```python
from build123d import *

# Parameters (mm, degrees)
F1_R     = 1.6
F1_W     = 26.4
F1_H     = 5
F1_W_2   = 20
F1_W_3   = 5
F2_DEPTH = 5


with BuildPart() as f2:
    # F1 (on Right) → F2 (new body)
    with BuildSketch(Plane.YZ):
        with BuildLine():
            Line((0, 5), (0, 0))
            Line((0, 0), (33.5, 0))
            Line((33.5, 0), (33.5, -5))
            Line((33.5, -5), (38.5, -5))
            Line((38.5, -5), (38.5, 0))
            Line((38.5, 0), (47, 0))
            Line((47, 0), (47, 2))
            Line((47, 2), (45.75, 2))
            Line((45.75, 2), (45.75, 5))
            Line((45.75, 5), (47, 5))
            Line((47, 5), (47, 6))
            Line((47, 6), (50, 6))
            Line((50, 6), (50, 5))
            Line((50, 5), (51.25, 5))
            Line((51.25, 5), (51.25, 2))
            Line((51.25, 2), (50, 2))
            Line((50, 2), (50, 0))
            Line((50, 0), (58.5, 0))
            Line((58.5, 0), (58.5, -5))
            Line((58.5, -5), (63.5, -5))
            Line((63.5, -5), (63.5, 0))
            Line((63.5, 0), (97, 0))
            Line((97, 0), (118.2132034356, -21.2132034356))
            Line((118.2132034356, -21.2132034356), (125.2842712475, -28.2842712475))
            Line((125.2842712475, -28.2842712475), (131.2239682094, -34.2239682094))
            Line((131.2239682094, -34.2239682094), (132.9917351624, -32.4562012565))
            Line((132.9917351624, -32.4562012565), (132.178562364, -31.6430284581))
            Line((132.178562364, -31.6430284581), (133.946329317, -29.8752615051))
            Line((133.946329317, -29.8752615051), (135.8908729653, -31.8198051534))
            Line((135.8908729653, -31.8198051534), (137.8354166135, -33.7643488017))
            Line((137.8354166135, -33.7643488017), (136.0676496606, -35.5321157546))
            Line((136.0676496606, -35.5321157546), (135.2544768622, -34.7189429563))
            Line((135.2544768622, -34.7189429563), (133.4867099092, -36.4867099092))
            Line((133.4867099092, -36.4867099092), (139.4264068712, -42.4264068712))
            Line((139.4264068712, -42.4264068712), (146.4974746831, -49.4974746831))
            Line((146.4974746831, -49.4974746831), (153.5685424949, -56.5685424949))
            Line((153.5685424949, -56.5685424949), (179.7314933988, -30.405591591))
            ThreePointArc((179.7314933988, -30.405591591), (180.6101730553, -28.2842712475), (179.7314933988, -26.1629509039))
            Line((179.7314933988, -26.1629509039), (110.8908729653, 42.6776695297))
            ThreePointArc((110.8908729653, 42.6776695297), (102.7802892447, 48.0969883128), (93.2132034356, 50))
            Line((93.2132034356, 50), (0, 50))
            Line((0, 50), (0, 35))
            Line((0, 35), (5, 35))
            Line((5, 35), (5, 30))
            Line((5, 30), (0, 30))
            Line((0, 30), (0, 10))
            Line((0, 10), (5, 10))
            Line((5, 10), (5, 5))
            Line((5, 5), (0, 5))
        make_face()
        with Locations((2.5, 20)):
            Circle(F1_R, mode=Mode.SUBTRACT)
        with Locations((40.6, 29.5)):
            Rectangle(F1_W, F1_H, mode=Mode.SUBTRACT)
        with Locations((48.5, 42.5)):
            Rectangle(F1_W_2, F1_H, mode=Mode.SUBTRACT)
        with Locations((94.5, 7.5)):
            Rectangle(F1_W_3, F1_H, mode=Mode.SUBTRACT)
        with Locations((94.5, 20)):
            Circle(F1_R, mode=Mode.SUBTRACT)
        with Locations((94.5, 32.5)):
            Rectangle(F1_W_3, F1_H, mode=Mode.SUBTRACT)
        Polygon((142.9619407771, -53.033008589), (146.4974746831, -49.4974746831), (139.4264068712, -42.4264068712), (135.8908729653, -45.9619407771), align=None)
        Polygon((125.2842712475, -28.2842712475), (118.2132034356, -21.2132034356), (114.6776695297, -24.7487373415), (121.7487373415, -31.8198051534), align=None)
    extrude(amount=F2_DEPTH)


solid = f2.part
```
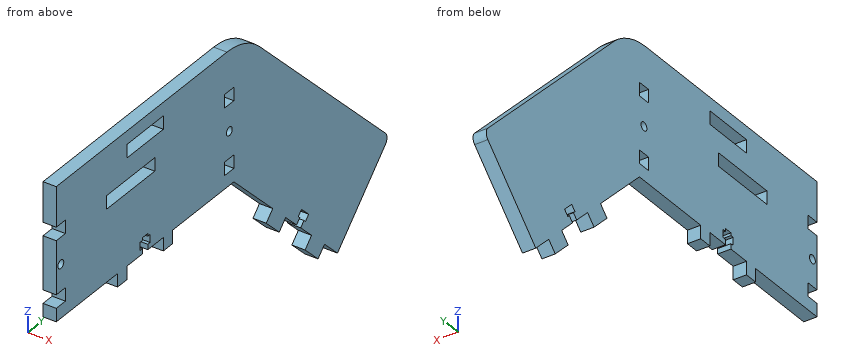
Model file for the job. Use its own axes, mm. Round coordinates to 2 decimals unless told otherwise and drop trailing zeros. Write each loop counter-clockwise with the first axis right and the second up, starting at its lowest first coordinate (ties: lowest second). Pieces come first, ordered by that corner, then holes. Notation, with made-up numbers: (5.25, 49.5) - (32.25, 49.5) arc R22 ccw to (32.25, 84.5) - close; hole circle Ø11 at (31.5, 41.25). An arc over 180 degrees is marked (long way). Use CSV: the item, a comma, the result in double quotes. Start each with the question number.
Item 1: Band-saw the part on B-B (y = 159.5). Write the cut outline in (x, z), and give its area (3 significant figures).
Item 2: Drill centre lines: L1, parallel to Z at x = 3.3, y = 94.5; L2, parallel to Z at x = 2.95, y = 40; L3, parallel to Z at x = 2.75, y = 36. Where is each one in solid material? Low to high. Write a range as [from, to].
Item 3: Pin check, flat tips, straight feed: P1, Ø1.5, axis at x = 2, y = 83.5, coming from the -Z side; P2, Ø1.5, axis at x = 1.5, z = 32, coming from the -Y side; P3, Ø3, axis at x = 1.5, z = -19.5, coming from the +Y side. Stop position of each tip, or through.
Item 4: Band-saw the part on A-A (x = 1.9). State how many separate pieces and enclosed holes the cut face has, and give its area (3 significant figures).
Checked values:
1,outline,"(0, -50.64) - (5, -50.64) - (5, -5.93) - (0, -5.93) - close"
1,area,"224 mm²"
2,L1,"z = [0, 5], [10, 18.4], [21.6, 30], [35, 49.97]"
2,L2,"z = [0, 27], [32, 40], [45, 50]"
2,L3,"z = [-5, 27], [32, 50]"
3,P1,"stops at z = 0"
3,P2,"stops at y = 5"
3,P3,"stops at y = 174.57"
4,separate pieces,"1"
4,enclosed holes,"6"
4,area,"8,570 mm²"
